Source: CAD feature listing. Evaluate the final solid. Frame: model axes, mm. Coordinates: 2 decimals unless noted, no trailing zeros. Order: outer loops, then holes, each group sorted by start corner. A loop starts at its lowest first (then second) coordinate and runs counter-clockwise, first axis right, second up.
```python
from build123d import *

# Parameters (mm, degrees)
F0_W     = 25.4
F0_H     = 76.2
F1_DEPTH = 7.62
F2_R     = 6.35
F3_DEPTH = 12.7
F5_DEPTH = 7.62
F6_R     = 3.81
F7_DEPTH = 7.62
F8_DEPTH = 5.08


with BuildPart() as f1:
    # F0 (on Top) → F1 (new body)
    with BuildSketch(Plane.XY):
        with Locations((-1.029531109, -3.4307520837)):
            Rectangle(F0_W, F0_H)
    extrude(amount=F1_DEPTH)

    # F2 (on face) → F3 (join)
    with BuildSketch(Plane(origin=(0, 0, 0), x_dir=(1, 0, 0), z_dir=(0, 0, -1))):
        with Locations((-1.029531109, -21.9692479163)):
            Circle(F2_R)
    extrude(amount=F3_DEPTH)

    # F4 (on face) → F5 (join)
    with BuildSketch(Plane(origin=(0, 0, 0), x_dir=(1, 0, 0), z_dir=(0, 0, -1))):
        with BuildLine():
            ThreePointArc((-13.729531109, -21.9692479163), (-13.6507066419, -20.5564746978), (-13.4152117126, -19.1612386598))
            add(Edge.make_bspline(
                [(-13.4152117126, -19.1612386598), (-12.8610433574, -14.3104636642), (-11.5717530157, -4.180075995), (-8.9574552779, 13.7376117238), (-1.3781278255, 26.6796034372), (5.8301842944, 35.8071219352), (11.670468891, 38.2592551099)],
                knots=[0.0402552104, 0.0402552104, 0.0402552104, 0.0402552104, 0.2518393979, 0.5131919232, 0.7477210565, 1, 1, 1, 1], degree=3))
            Line((11.670468891, 38.2592551099), (11.670468891, 41.5307520837))
            Line((11.670468891, 41.5307520837), (-13.729531109, 41.5307520837))
            Line((-13.729531109, 41.5307520837), (-13.729531109, -21.9692479163))
        make_face()
    extrude(amount=F5_DEPTH)

    # F6 (on face) → F7 (cut)
    with BuildSketch(Plane(origin=(0, 0, -7.62), x_dir=(1, 0, 0), z_dir=(0, 0, -1))):
        with BuildLine():
            Line((-13.729531109, 41.5307520837), (-13.729531109, -21.9692479163))
            ThreePointArc((-13.729531109, -21.9692479163), (-13.6507066419, -20.5564746978), (-13.4152117126, -19.1612386598))
            add(Edge.make_bspline(
                [(-13.4152117126, -19.1612386598), (-12.8610433574, -14.3104636642), (-11.5717530157, -4.180075995), (-8.9574552779, 13.7376117238), (-1.3781278255, 26.6796034372), (5.8301842944, 35.8071219352), (11.670468891, 38.2592551099)],
                knots=[0.0402552104, 0.0402552104, 0.0402552104, 0.0402552104, 0.2518393979, 0.5131919232, 0.7477210565, 1, 1, 1, 1], degree=3))
            Line((11.670468891, 38.2592551099), (11.670468891, 41.5307520837))
            Line((11.670468891, 41.5307520837), (-13.729531109, 41.5307520837))
        make_face()
        with Locations((-7.379531109, 35.1807520837)):
            Circle(F6_R, mode=Mode.SUBTRACT)
    extrude(amount=-F7_DEPTH, mode=Mode.SUBTRACT)

    # F8 (add): a face of the model
    f8_faces = [f1.faces().sort_by_distance(p)[0] for p in [
        (-7.379531109, -35.1807520837, -7.62),
    ]]
    extrude(f8_faces, amount=F8_DEPTH)


solid = f1.part
```
Q1. Material intervals for line 1 along Z through (x, y) = (-11, -17); line 2 along Y through (x, z) = (-1, -11.5); line 3 along Y through (x, z) = (-9, -1.5), sorted ascending.
Solutions:
line 1: z = 0 to 7.62
line 2: y = 15.62 to 28.32
line 3: y = -38.63 to -31.73
Q2. Section query D-D on y = 20.5. Output: boundary loops of the cut face in (x, z).
Solutions:
outline: (-13.73, 0) - (-7.21, 0) - (-7.21, -12.7) - (5.15, -12.7) - (5.15, 0) - (11.67, 0) - (11.67, 7.62) - (-13.73, 7.62) - close
Q3. Section query C-C on z = -5.5. Output: boundary loops of the cut face in (x, y).
Solutions:
outline: circle Ø7.62 at (-7.38, -35.18); circle Ø12.7 at (-1.03, 21.97)
Q4. Section query A-A on y = -34. Output: boundary loops of the cut face in (x, z), plus the area to 3 significant figures.
Solutions:
outline: (-13.73, 0) - (-11, 0) - (-11, -12.7) - (-3.76, -12.7) - (-3.76, 0) - (11.67, 0) - (11.67, 7.62) - (-13.73, 7.62) - close
area: 286 mm2
Q5. Pull-direction query (Y, two-part tool) for faces 1 (the flat face through (-1, 34.669, 4)), 2 (the flat face through (-1, 22, -12.7)), 3 (the flat face through (-1, -41.531, 4)), 4 (the cylindrical face through (1.901, 27.603, -6.261)); classes: pulls with the +Y half, pulls with the -Y half, needs draft (parallel to the pull), parting line crosses it, or undercut.
Solutions:
face 1: pulls with the +Y half
face 2: needs draft
face 3: pulls with the -Y half
face 4: undercut
Q6. Pin query (flat end, axial travel): P1, Ø4, axis at y = -33.5, z = -7.5, coming from the -X side; P2, Ø8, axis at x = -3, z = -6, coming from the +Y side; P3, Ø3, axis at x = 0.5, y = 0, coming from the -Z side; P4, Ø1, axis at y = 14.5, z = -6.5, coming from the +X side. Return the tip coordinate at first contact, or that it passes through.
Solutions:
P1: stops at x = -11.19
P2: stops at y = 28.32
P3: stops at z = 0
P4: passes through
Q7. Section query B-B on x = 6. Output: boundary loops of the cut face in (y, z).
Solutions:
outline: (-41.53, 0) - (34.67, 0) - (34.67, 7.62) - (-41.53, 7.62) - close
